Autodesk Inventor part; units mm, degrees
ref_plane "YZ Plane" through (0, 0, 0) normal (1, 0, 0) x (0, 1, 0)
ref_plane "XZ Plane" through (0, 0, 0) normal (0, 1, 0) x (-1, 0, 0)
ref_plane "XY Plane" through (0, 0, 0) normal (0, 0, 1) x (1, 0, 0)
sketch "草图1" plane through (0, 0, 0) normal (0, 0, 1) x (1, 0, 0)
  circle A0 centre (-95, 67.5) radius 25
  circle A1 centre (0, 0) radius 20
  line L0 (-79.6588, 87.2395) -> (12.273, 15.7916)
  line L1 (-108.5925, 46.518) -> (-10.874, -16.7856)
  line L2 (-77.511, 90.003) -> (14.4207, 18.5551)
  line L3 (-110.4954, 43.5805) -> (-12.7769, -19.7231)
  arc A2 (-77.511, 90.003) -> (-110.4954, 43.5805) centre (-95, 67.5) ccw
  arc A3 (-12.7769, -19.7231) -> (14.4207, 18.5551) centre (0, 0) ccw
  dimension "d0" = 50
  dimension "d1" = 40
  dimension "d2" = 95
  dimension "d3" = 67.5
  dimension "d4" = 3.5
  dimension "d5" = 3.5
extrude "拉伸1" add sketch "草图1" along normal blind 15.423
chamfer "倒角1" distance 3.5 distance2 2.021 4 edges at (16.3036, -11.5841, 15.423) (-59.7332, 14.8662, 15.423) (-115.3795, 81.9802, 15.423) (-33.6929, 51.5155, 15.423) measured on face at (-16.9391, 41.4499, 15.423)
chamfer "倒角2" distance 3.5 distance2 2.021 4 edges at (-59.7332, 14.8662, 0) (16.3036, -11.5841, 0) (-33.6929, 51.5155, 0) (-115.3795, 81.9802, 0) measured on face at (-16.9391, 41.4499, 0)
properties part number "砂轮皮带"
Here's how the part is built. I have some questions about the finished solid (model axes, mm). A direction names the side the tool comes from. Coordinates: 2 decimals unless noted, no trailing zeros. Loops run counter-clockwise (first coordinate to the right, second up) from the corner with the lowest first, then second, coordinate; pieces in that order, holes last. Notation, with made-up numbers: (51, 1) -> (70, 1) arc R27 ccw to (70, 27) -> close; hole circle Ø11 at (56, 55.25). An arc over 180 degrees is marked (long way). Use one line per item in the form item = value. Start each with the question number.
(1) We'd pull the mould along X, two halves only. Please class faces 1 (the face through (19.443, -13.199, 7.604)), 2 (the face through (16.23, -12.06, 13.53)), 3 (the face through (-62.32, 12.37, 7.6)): pulls with the +X half, pulls with the -X half, needs draft (parallel to the pull), parting line crosses it, or undercut.
(2) Please list where these lines run through material, in increasing order: line 1 along Y through (x, z) = (10, 6.75); line 2 along Y through (x, z) = (-96.5, 13.5); line 3 along X through (y, z) = (49.5, 8.5).
(3) Will these pins go through, and if not, where does the flat tip stop? pin 1 (6 mm diameter, centred on y = 22.5, z = 4.5, fed in from +X); pin 2 (8 mm diameter, centred on x = -78.5, y = 82, fed in from -Z); pin 3 (4 mm diameter, centred on y = -3.5, z = 9, fed in from +X).
(4) On a 3-axis mill with a long thin cutter (end or side, diameter ignored), from which of +Z, -Z, +X, -X, +Y, -Y can I reach the whole of each face in a straight line? I mean faces 4 (the face through (-61.355, 13.861, 1.025)), 5 (the face through (-34.34, 52.02, 7.63)), 6 (the face through (-33.3, 53.4, 14.4)), 7 (the face through (-32.19, 54.78, 7.6)). Say none if no direction works.
(5) If we section it at C-C (z = 5): Please give me the cut outline in (x, y).
Verdict:
q1.face_1 = parting line crosses it
q1.face_2 = undercut
q1.face_3 = pulls with the -X half
q2.line_1 = -21.27 to -17.32, 17.56 to 21.99
q2.line_2 = 34.51 to 38.48, 92.62 to 95.96
q2.line_3 = -117.1 to -112.35, -31.1 to -25.4
q3.pin_1 = 13.2
q3.pin_2 = 1.69
q3.pin_3 = 23.45
q4.face_4 = -Z
q4.face_5 = +Z, -Z
q4.face_6 = +Z
q4.face_7 = +Z, -Z, +X, +Y
q5.outline = (-110.5, 43.58) -> (-12.78, -19.72) arc R23.5 ccw to (14.42, 18.56) -> (-77.51, 90) arc R28.5 ccw (long way) to start; hole (-108.59, 46.52) -> (-10.87, -16.79) arc R20 ccw to (12.27, 15.79) -> (-79.66, 87.24) arc R25 ccw (long way) to start
